from build123d import *

# Parameters (mm, degrees)
SKETCH_1_W      = 22
SKETCH_1_H      = 55
EXTRUDE_1_DEPTH = 2
SKETCH_2_W      = 2.2
SKETCH_2_H      = 52
EXTRUDE_2_DEPTH = 10
SKETCH_4_W      = 8
SKETCH_4_H      = 5
EXTRUDE_3_DEPTH = 8


with BuildPart() as part:
    # 草图1 → 凸台-拉伸1 (new body)
    with BuildSketch(Plane.XY):
        Rectangle(SKETCH_1_W, SKETCH_1_H)
    extrude(amount=EXTRUDE_1_DEPTH)

    # 草图2 → 凸台-拉伸2 (add)
    with BuildSketch(Plane.XY):
        with Locations((8, 0)):
            Rectangle(SKETCH_2_W, SKETCH_2_H)
        with Locations((-8, 0)):
            Rectangle(SKETCH_2_W, SKETCH_2_H)
    extrude(amount=-EXTRUDE_2_DEPTH)

    # 草图4 → 凸台-拉伸3 (add)
    with BuildSketch(Plane.XY.offset(2)):
        with Locations((0, 18)):
            Rectangle(SKETCH_4_W, SKETCH_4_H)
    extrude(amount=EXTRUDE_3_DEPTH)


solid = part.part
Source: CAD feature listing. Evaluate the final solid. Frame: model axes, mm. A direction names the side the tool comes from. Give positions to 0.01 mm unless a question says otherwise; leave off trailing zeros. Loops run counter-clockwise (first coordinate to the right, second up) from the corner with the lowest first, then second, coordinate; pieces in that order, holes last. Notation, with made-up numbers: (-22.5, -11) -> (8.5, -11) arc R9 ccw to (8.5, -2) -> close; hole circle Ø6 at (-5.5, 8.5). An arc over 180 degrees is marked (long way). Use a Markdown table: item, result. Add a question column.
1) Section query D-D, the plane y = 18. Return the cut outline in (x, z).
2) Pull-direction query (X, two-part tool) for faces 4 (the face through (0, 15.5, 6)), 5 (the face through (11, 0, 1)), 6 (the face through (0, 0, 0)); classes: +X half, -X half, draft (parallel to the pull), parting line (faces both ways), or undercut.
3) Section query C-C, the plane x = 1.25. Return the cut outline in (y, z).
4) Section query A-A, the plane z = -3.25. Return the cut outline in (x, y).
5) Line query: line 1 along X through (y, z) = (11.5, -5); line 2 along Z through (x, y) = (-10, 23.5); line 3 along Y through (x, z) = (-3, 2.5). Output: solid intervals per line, ascending. Write a range as [from, to].
6) First-contact query: pin 1 (0.7 mm diameter, centred on x = -8, z = -2.5, fed in from -Y); pin 2 (3 mm diameter, centred on y = 8, z = -3.5, fed in from -X); pin 3 (1.1 mm diameter, centred on x = -8, z = -3, fed in from +Y). Flat tips, straight axial feed; report the tip coordinate or a pass-through.
7) Section query B-B, the plane y = -8. Return the cut outline in (x, z), then the cut area to 3 significant figures.
8) Reachability of faces 1 (the face through (-8, -26, -5)), 2 (the face through (-8, 26, -5)), 3 (the face through (6.9, 0, -5)) from +Z, -Z, +X, -X, +Y, -Y: full face, straight path, thin tool, end or side. Return the list, or none.
Numbers:
| question | item | result |
|---|---|---|
| 1 | outline | (-11, 0) -> (-9.1, 0) -> (-9.1, -10) -> (-6.9, -10) -> (-6.9, 0) -> (6.9, 0) -> (6.9, -10) -> (9.1, -10) -> (9.1, 0) -> (11, 0) -> (11, 2) -> (4, 2) -> (4, 10) -> (-4, 10) -> (-4, 2) -> (-11, 2) -> close |
| 2 | face 4 | draft |
| 2 | face 5 | +X half |
| 2 | face 6 | undercut |
| 3 | outline | (-27.5, 0) -> (27.5, 0) -> (27.5, 2) -> (20.5, 2) -> (20.5, 10) -> (15.5, 10) -> (15.5, 2) -> (-27.5, 2) -> close |
| 4 | outline | (-9.1, -26) -> (-6.9, -26) -> (-6.9, 26) -> (-9.1, 26) -> close; (6.9, -26) -> (9.1, -26) -> (9.1, 26) -> (6.9, 26) -> close |
| 5 | line 1 | x = [-9.1, -6.9], [6.9, 9.1] |
| 5 | line 2 | z = [0, 2] |
| 5 | line 3 | y = [15.5, 20.5] |
| 6 | pin 1 | stops at y = -26 |
| 6 | pin 2 | stops at x = -9.1 |
| 6 | pin 3 | stops at y = 26 |
| 7 | outline | (-11, 0) -> (-9.1, 0) -> (-9.1, -10) -> (-6.9, -10) -> (-6.9, 0) -> (6.9, 0) -> (6.9, -10) -> (9.1, -10) -> (9.1, 0) -> (11, 0) -> (11, 2) -> (-11, 2) -> close |
| 7 | area | 88.0 mm2 |
| 8 | face 1 | -Z, +X, -X, -Y |
| 8 | face 2 | -Z, +X, -X, +Y |
| 8 | face 3 | -Z, +Y, -Y |
